The drawing under review shows one solid part. Ordinate dimensions are in mm from its lowest x, y, z. A direction names the side the tool comes from. Coordinates: 2 decimals unless noted, no trailing zeros. Write each loop counter-clockwise with the first axis right and the second up, starting at its lowest first coordinate (ties: lowest second). Pieces come first, ordered by that corner, then holes. Notation, with made-up numbers: (34.5, -26) -> (80.5, -26) arc R20 ccw to (80.5, -2) -> close; hole circle Ø5 at (59.25, 22). An arc over 180 degrees is marked (long way). One line per item, written item: value. Start each with the question number.
1) Add section A-A (y = 3). State the section outline as (x, z) points, and give its area (3 significant figures).
2) Machinability: for the marked faces 1 and 2, which of the approach directions +Z, -Z, +X, -X, +Y, -Y give a long, thin tool a straight path to every point of the face, cutting with its end or side? Answer none if there is none.
3) Add section D-D (x = 0.5). State the section outline as (y, z) points, and give its area (3 significant figures).
4) For probe 1 along Y at (x, z) = (3, 5.5); probe 2 along Z at (x, y) = (4.35, 5.2); probe 3 along Y at (x, z) = (2.3, 2.75), list the stretches that pass through material, from the lowest coordinate up. Write a range as from..to.
5) Add section C-C (z = 1.75). State the section outline as (x, y) points, and give its area (3 significant figures).
6) For pin 1 Ø1.5 at (y, z) = (4.5, 2) entering from +X; pin 2 Ø1.5 at (x, z) = (2, 4) entering from +Y, all flat-tipped, find the tip position at first contact; note any pin that passes through.
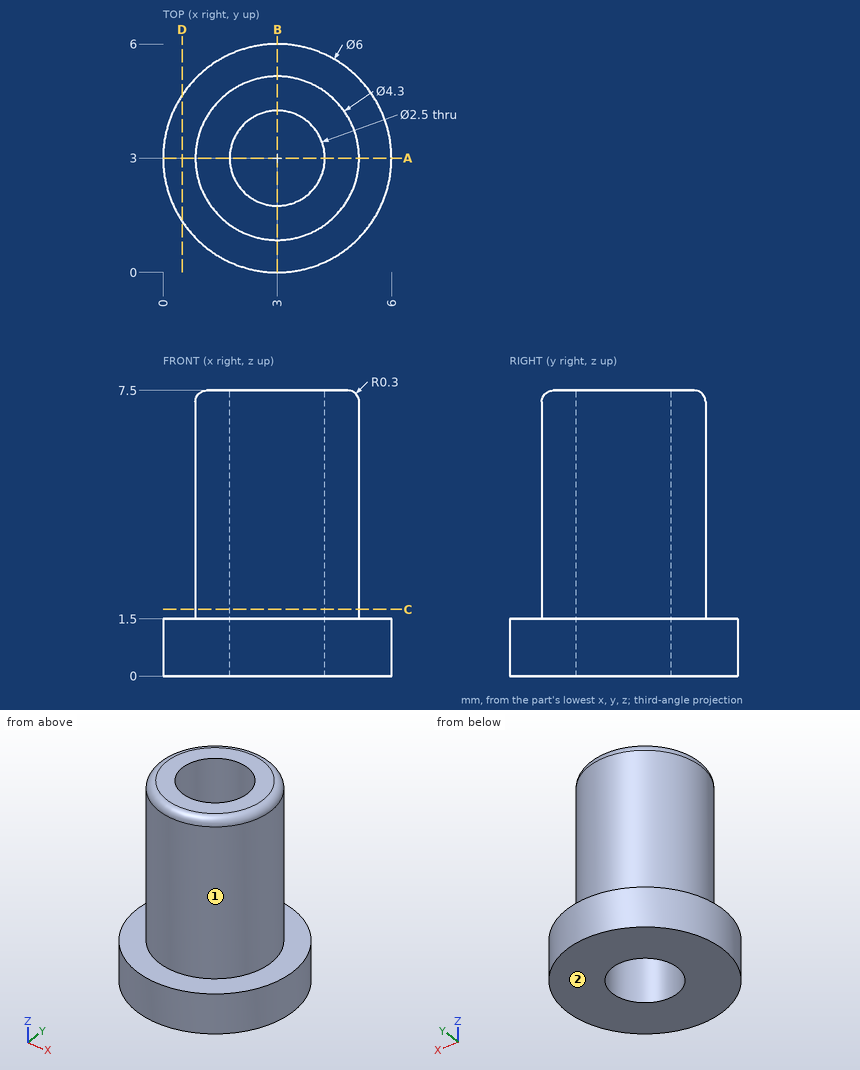
Numbers:
1. outline: (0, 0) -> (1.75, 0) -> (1.75, 7.5) -> (1.15, 7.5) arc R0.3 ccw to (0.85, 7.2) -> (0.85, 1.5) -> (0, 1.5) -> close; (4.25, 0) -> (6, 0) -> (6, 1.5) -> (5.15, 1.5) -> (5.15, 7.2) arc R0.3 ccw to (4.85, 7.5) -> (4.25, 7.5) -> close
1. area: 16.0 mm²
2. face 1: +Z
2. face 2: -Z, +X, -X, +Y, -Y
3. outline: (1.34, 0) -> (4.66, 0) -> (4.66, 1.5) -> (1.34, 1.5) -> close
3. area: 4.97 mm²
4. probe 1: 0.85..1.75, 4.25..5.15
4. probe 2: 0..1.5
4. probe 3: 0.97..1.96, 4.04..5.03
5. outline: circle Ø4.3 at (3, 3); hole circle Ø2.5 at (3, 3)
5. area: 9.61 mm²
6. pin 1: x = 5.85
6. pin 2: y = 5.14
